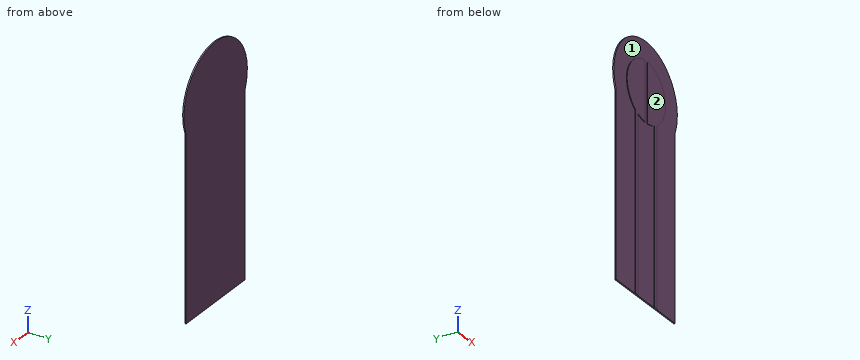
```python
from build123d import *

# Parameters (mm, degrees)
F1_DEPTH = 0.1
F3_DEPTH = 0.05


with BuildPart() as f1:
    # F0 (on Front) → F1 (new body)
    with BuildSketch(Plane.XZ):
        with BuildLine():
            Line((-3.555, -7.811804), (3.555, -7.811804))
            Line((3.555, -7.811804), (3.555, 6.441375))
            ThreePointArc((3.555, 6.441375), (0, 11.621804), (-3.555, 6.441375))
            Line((-3.555, 6.441375), (-3.555, -7.811804))
        make_face()
    extrude(amount=F1_DEPTH)

    # F2 (on face) → F3 (join)
    with BuildSketch(Plane.XZ.offset(0.1)):
        with BuildLine():
            Line((-0.141701, 5.516975), (-0.141713, 10.106631))
            ThreePointArc((-0.141713, 10.106631), (-2.216193, 8.424019), (-1.2996, 5.915133))
            Line((-1.2996, 5.915133), (-1.2996, -7.811803))
            Line((-1.2996, -7.811803), (-0.9996, -7.811803))
            Line((-0.9996, -7.811803), (-0.9996, 5.741268))
            ThreePointArc((-0.9996, 5.741268), (-0.581566, 5.587371), (-0.141701, 5.516975))
        make_face()
        with BuildLine():
            ThreePointArc((1.2996, 5.915133), (2.216191, 8.424025), (0.141701, 10.106632))
            Line((0.141701, 10.106632), (0.141713, 5.516976))
            ThreePointArc((0.141713, 5.516976), (0.581571, 5.587373), (0.9996, 5.741268))
            Line((0.9996, 5.741268), (0.9996, -7.811803))
            Line((0.9996, -7.811803), (1.2996, -7.811803))
            Line((1.2996, -7.811803), (1.2996, 5.915133))
        make_face()
    extrude(amount=F3_DEPTH)


solid = f1.part
```
Model file for the job. Use its own axes, mm. Face numbers are marked on the shaded views. Give positions to 0.01 mm unless a question says otherwise; leave off trailing zeros. Write each loop counter-clockwise with the first axis right and the second up, starting at its lowest first coordinate (ties: lowest second). Pieces come first, ordered by that corner, then holes. Notation, with made-up numbers: (17.25, -8.75) - (24.25, -8.75) arc R31 cw to (24.25, 30.25) - close; hole circle Ø10 at (-17.75, -31.75). An arc over 180 degrees is marked (long way). One line per question, with ' | ' between items. Start each with the question number.
(1) Slice it at C-C on x = -1.5. Write the cut outline in (y, z).
(2) Slice it at B-B on y = -0.05. Write the cut outline in (x, z) (3 decimals), plus the area to 3 significant figures.
(3) Slice it at A-A on z = 7. Write the cut outline in (x, y), plus the area to 3 significant figures.
(4) Two-plate mould, pull along X, no slides. Class the marked faces 1 and 2: +X half, -X half, draft (parallel to the pull), parting line (faces both ways), or undercut.
(5) Wall check: line 1 along X through (y, z) = (-0.05, 5.75) (3 decimals); line 2 along Z through (x, y) = (1.25, -0.05); line 3 along Z through (x, y) = (-3, -0.05). Give the ranges that are in metal, low to high. Write a range as from..to.
(6) Slice it at D-D on x = -3. Write the cut outline in (y, z).
Results below:
1) outline: (-0.15, 6.07) - (-0.1, 6.07) - (-0.1, -7.81) - (0, -7.81) - (0, 11.31) - (-0.1, 11.31) - (-0.1, 9.55) - (-0.15, 9.55) - close
2) outline: (-3.555, -7.812) - (3.555, -7.812) - (3.555, 6.441) arc R3.81 ccw (long way) to (-3.555, 6.441) - close | area: 134 mm^2
3) outline: (-3.72, -0.1) - (-2.15, -0.1) - (-2.15, -0.15) - (-0.14, -0.15) - (-0.14, -0.1) - (0.14, -0.1) - (0.14, -0.15) - (2.15, -0.15) - (2.15, -0.1) - (3.72, -0.1) - (3.72, 0) - (-3.72, 0) - close | area: 0.945 mm^2
4) face 1: undercut | face 2: draft
5) line 1: -3.555..3.555 | line 2: -7.81..11.41 | line 3: -7.81..10.16
6) outline: (-0.1, -7.81) - (0, -7.81) - (0, 10.16) - (-0.1, 10.16) - close
